For this review, use the dimensioned drawing (mm, ordinates from the lowest corner) and the shaded views. A direction names the side the tool comes from. Round coordinates to 2 decimals unless told otherwise and drop trailing zeros. Write each loop counter-clockwise with the first axis right and the second up, starting at its lowest first coordinate (ties: lowest second). Pieces come first, ordered by that corner, then holes. Notation, with made-up numbers: M 47,42.25 L 59,42.25 A27 cw 59,59.25 Z; hole C 22,10 d6. An arc over 180 degrees is marked long. One line per question, with ' | ' between items. Start each with the question number.
Item 1: For L1, parallel to X at y = 61, z = 19; L2, parallel to X at y = 40, z = 33 (1 decimal); L3, parallel to Y at x = 1.45, z = 19.05, list the stretches that pass through material, from the lowest coordinate up.
Item 2: Add section A-A, the plane z = 19.05. State the section outline as (x, y) points (1 decimal), and give its area (3 significant figures).
Item 3: Add section D-D, the plane z = 31. State the section outline as (x, y) points (1 decimal).
Item 4: Add section C-C, the plane z = 35. State the section outline as (x, y) points (1 decimal).
Item 5: Insertion check: pin 1 Ø5 at (x, z) = (27, 25) entering from -Y (3 decimals). The pin has a flat end and moves straight along its axis. Give the tip position at first contact, or say it passes through.
Item 6: Add section B-B, the plane y = 46.5. State the section outline as (x, z) points (1 decimal), and give its area (3 significant figures).
Item 7: Draft analysis for pull direction X (two halves, no side actions). For the marked faces 3, 4 and 5, state which applies: released by +X, released by -X, zero draft, split by the parting line, or undercut.
Item 8: Machinability: for the marked faces 1 and 2, which of the approach directions +Z, -Z, +X, -X, +Y, -Y give a long, thin tool a straight path to every point of the face, cutting with its end or side? Answer none if there is none.
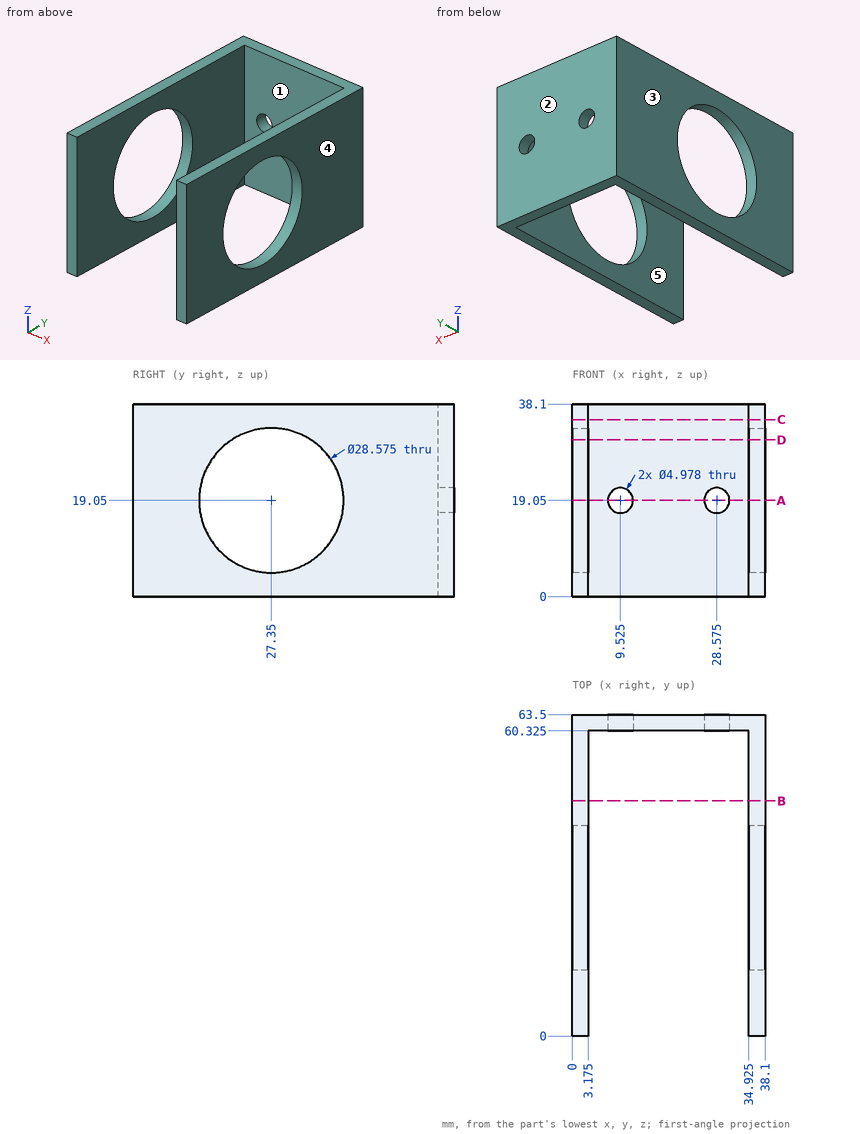
Computed values:
1) L1: x = 0 to 7.04, 12.01 to 26.09, 31.06 to 38.1 | L2: x = 0 to 3.2, 34.9 to 38.1 | L3: y = 0 to 13.06, 41.64 to 63.5
2) outline: M 0,0 L 3.2,0 L 3.2,13.1 L 0,13.1 Z; M 0,41.6 L 3.2,41.6 L 3.2,60.3 L 7,60.3 L 7,63.5 L 0,63.5 Z; M 12,60.3 L 26.1,60.3 L 26.1,63.5 L 12,63.5 Z; M 31.1,60.3 L 34.9,60.3 L 34.9,41.6 L 38.1,41.6 L 38.1,63.5 L 31.1,63.5 Z; M 34.9,0 L 38.1,0 L 38.1,13.1 L 34.9,13.1 Z | area: 291 mm^2
3) outline: M 0,0 L 3.2,0 L 3.2,19.5 L 0,19.5 Z; M 0,35.2 L 3.2,35.2 L 3.2,60.3 L 34.9,60.3 L 34.9,35.2 L 38.1,35.2 L 38.1,63.5 L 0,63.5 Z; M 34.9,0 L 38.1,0 L 38.1,19.5 L 34.9,19.5 Z
4) outline: M 0,0 L 3.2,0 L 3.2,60.3 L 34.9,60.3 L 34.9,0 L 38.1,0 L 38.1,63.5 L 0,63.5 Z
5) pin 1: stops at y = 60.325
6) outline: M 0,0 L 3.2,0 L 3.2,38.1 L 0,38.1 Z; M 34.9,0 L 38.1,0 L 38.1,38.1 L 34.9,38.1 Z | area: 242 mm^2
7) face 3: released by -X | face 4: released by +X | face 5: undercut
8) face 1: +Z, -Z, -Y | face 2: +Z, -Z, +X, -X, +Y
